from build123d import *

# Parameters (mm, degrees)
SKETCH1_W            = 73.66
SKETCH1_H            = 69.85
BOSS_EXTRUDE1_DEPTH  = 8.89
SKETCH2_R            = 2.032
CUT_EXTRUDE1_DEPTH   = 8.89
SKETCH3_W            = 73.66
SKETCH3_H            = 6.35
BOSS_EXTRUDE2_DEPTH  = 127
SKETCH4_W            = 73.66
SKETCH4_H            = 6.35
BOSS_EXTRUDE3_DEPTH  = 38.1
BOSS_EXTRUDE4_START  = -36.83
BOSS_EXTRUDE4_DEPTH  = 6.35
SKETCH7_R            = 2.54
SKETCH7_R_2          = 6.35
CUT_EXTRUDE2_DEPTH   = 6.35
BOSS_EXTRUDE15_DEPTH = 12.7
SKETCH23_R           = 6.35
BOSS_EXTRUDE16_DEPTH = 6.35
BOSS_EXTRUDE17_DEPTH = 12.7
SKETCH25_W           = 27.94
SKETCH25_H           = 6.35
BOSS_EXTRUDE18_DEPTH = 6.35


with BuildPart() as part:
    # Sketch1 → Boss-Extrude1 (new body)
    with BuildSketch(Plane.XY):
        Rectangle(SKETCH1_W, SKETCH1_H)
    extrude(amount=BOSS_EXTRUDE1_DEPTH)

    # Sketch2 → Cut-Extrude1 (cut)
    with BuildSketch(Plane(origin=(0, 0, 0), x_dir=(-1, 0, 0), z_dir=(0, 0, -1))):
        with Locations((-29.9085, 26.035)):
            Circle(SKETCH2_R)
        with Locations((-29.9085, 8.255)):
            Circle(SKETCH2_R)
        with Locations((29.9085, 8.255)):
            Circle(SKETCH2_R)
        with Locations((29.9085, 26.035)):
            Circle(SKETCH2_R)
    extrude(amount=-CUT_EXTRUDE1_DEPTH, mode=Mode.SUBTRACT)

    # Sketch3 → Boss-Extrude2 (add)
    with BuildSketch(Plane(origin=(0, 0, 0), x_dir=(-1, 0, 0), z_dir=(0, 0, -1))):
        with Locations((0, -31.75)):
            Rectangle(SKETCH3_W, SKETCH3_H)
    extrude(amount=BOSS_EXTRUDE2_DEPTH)

    # Sketch4 → Boss-Extrude3 (add)
    with BuildSketch(Plane.XY.offset(8.89)):
        with Locations((0, -31.75)):
            Rectangle(SKETCH4_W, SKETCH4_H)
    extrude(amount=BOSS_EXTRUDE3_DEPTH)

    # Sketch5 → Boss-Extrude4 (add, symmetric)
    with BuildSketch(Plane(origin=(36.83, 0, 0), x_dir=(0, 0, -1), z_dir=(1, 0, 0)).offset(BOSS_EXTRUDE4_START)):
        Polygon((-46.99, -28.575), (-8.89, 25.837439057), (-8.89, -28.575), align=None)
    extrude(amount=BOSS_EXTRUDE4_DEPTH, both=True)

    # Sketch7 → Cut-Extrude2 (cut)
    with BuildSketch(Plane(origin=(0, -28.575, 0), x_dir=(1, 0, 0), z_dir=(0, 1, 0))):
        with Locations((0, 26.416)):
            Circle(SKETCH7_R)
        with Locations((0, 89.916)):
            Circle(SKETCH7_R_2)
    extrude(amount=-CUT_EXTRUDE2_DEPTH, mode=Mode.SUBTRACT)

    # Sketch21 → Boss-Extrude15 (add)
    with BuildSketch(Plane.ZY.offset(36.83)):
        Polygon((-25.4, -28.575), (-55.626, 3.175), (-49.276, 3.175), (-49.276, 9.525), (-13.0048, -28.575), align=None)
    extrude(amount=-BOSS_EXTRUDE15_DEPTH)

    # Sketch23 → Boss-Extrude16 (add)
    with BuildSketch(Plane(origin=(0, 3.175, 0), x_dir=(1, 0, 0), z_dir=(0, 1, 0))):
        with BuildLine():
            Line((-36.83, 49.276), (8.89, 49.276))
            Line((8.89, 49.276), (8.89, 89.916))
            ThreePointArc((8.89, 89.916), (0, 98.806), (-8.89, 89.916))
            Line((-8.89, 89.916), (-8.89, 55.626))
            Line((-8.89, 55.626), (-36.83, 55.626))
            Line((-36.83, 55.626), (-36.83, 49.276))
        make_face()
        with Locations((0, 89.916)):
            Circle(SKETCH23_R, mode=Mode.SUBTRACT)
    extrude(amount=BOSS_EXTRUDE16_DEPTH)

    # Sketch24 → Boss-Extrude17 (add)
    with BuildSketch(Plane(origin=(36.83, 0, 0), x_dir=(0, 0, -1), z_dir=(1, 0, 0))):
        Polygon((25.4, -28.575), (55.626, 3.175), (49.276, 3.175), (49.276, 9.525), (13.0048, -28.575), align=None)
    extrude(amount=-BOSS_EXTRUDE17_DEPTH)

    # Sketch25 → Boss-Extrude18 (add)
    with BuildSketch(Plane(origin=(0, 3.175, 0), x_dir=(1, 0, 0), z_dir=(0, 1, 0))):
        with Locations((22.86, 52.451)):
            Rectangle(SKETCH25_W, SKETCH25_H)
    extrude(amount=BOSS_EXTRUDE18_DEPTH)


solid = part.part
Design review of the part built by this model. Coordinates are the model's own, in mm. A direction names the side the tool comes from. Round coordinates to 2 decimals unless told otherwise and drop trailing zeros. Write each loop counter-clockwise with the first axis right and the second up, starting at its lowest first coordinate (ties: lowest second). Pieces come first, ordered by that corner, then holes. Notation, with made-up numbers: (70.5, -24) -> (105.5, -24) arc R16 cw to (105.5, -14) -> close; hole circle Ø10 at (-11, 33). An arc over 180 degrees is marked (long way). One line per question, with ' | ' between items.
(1) Insertion check: P1, Ø2.5, axis at x = 29.91, y = 26.04, coming from the -Z side; P2, Ø5.5, axis at x = 29.91, y = 8.26, coming from the -Z side; P3, Ø6.5, axis at x = -29.91, y = 26.04, coming from the -Z side; P4, Ø1.5, axis at x = 5.5, y = 6.5, coming from the -Z side. Each pin has a flat end and moves straight along its axis. Give the tip position at first contact, or say it passes through.
Result sheet:
P1: through | P2: z = -55.63 | P3: z = 0 | P4: z = -97.43
(2) Take a section at C-C, the plane y = -3. State the section outline as (x, z) points.
Result sheet:
outline: (-36.83, -49.75) -> (-24.13, -49.75) -> (-24.13, -37.35) -> (-36.83, -37.35) -> close; (-36.83, 0) -> (36.83, 0) -> (36.83, 8.89) -> (6.35, 8.89) -> (6.35, 29.08) -> (-6.35, 29.08) -> (-6.35, 8.89) -> (-36.83, 8.89) -> close; (24.13, -49.75) -> (36.83, -49.75) -> (36.83, -37.35) -> (24.13, -37.35) -> close
(3) Machinability: for faces 4 (the flat face through (23, 6, -55.626)), 5 (the flat face through (-1, 4, 0)), 6 (the flat face through (6.35, -13, 19)), 7 (the flat face through (-22, -28.575, 28)), 8 (the cylindrical face through (-31.847, 8.865, 4.383)), which of the approach directions +Z, -Z, +X, -X, +Y, -Y give a long, thin tool a straight path to every point of the face, cutting with its end or side? Answer none if there is none.
Result sheet:
face 4: -Z, +X, +Y | face 5: +X, -X, +Y | face 6: +Z, +X, +Y | face 7: +Z, -X, +Y | face 8: +Z
(4) Wall thickness on line 1 (Z direction, x = 0, y = -30.25); line 2 (Z direction, x = 0, y = 8.25); line 3 (Y direction, x = 7.5, z = -3) (3 decimals): over which ranges is each line inside the solid? List them lowest first. Write a range as [from, to].
Result sheet:
line 1: [-127, -96.27], [-83.57, -28.96], [-23.88, 46.99] | line 2: [-98.81, -96.27], [-83.57, -49.28], [0, 21.2] | line 3: [-34.925, -28.575]
(5) Take a section at A-A, the plane z = -61. State the section outline as (x, y) points (3 decimals).
Result sheet:
outline: (-36.83, -34.925) -> (36.83, -34.925) -> (36.83, -28.575) -> (-36.83, -28.575) -> close; (-8.89, 3.175) -> (8.89, 3.175) -> (8.89, 9.525) -> (-8.89, 9.525) -> close
(6) Take a section at D-D, the plane x = -22.5. State the section outline as (y, z) points (3 decimals), and give its area (3 significant figures).
Result sheet:
outline: (-34.925, -127) -> (-28.575, -127) -> (-28.575, 0) -> (34.925, 0) -> (34.925, 8.89) -> (-28.575, 8.89) -> (-28.575, 46.99) -> (-34.925, 46.99) -> close; (3.175, -55.626) -> (9.525, -55.626) -> (9.525, -49.276) -> (3.175, -49.276) -> close | area: 1,710 mm2
(7) Take a section at B-B, the plane x = 0. State the section outline as (y, z) points (3 decimals).
Result sheet:
outline: (-34.925, -127) -> (-28.575, -127) -> (-28.575, -96.266) -> (-34.925, -96.266) -> close; (-34.925, -83.566) -> (-28.575, -83.566) -> (-28.575, -28.956) -> (-34.925, -28.956) -> close; (-34.925, -23.876) -> (-28.575, -23.876) -> (-28.575, 0) -> (34.925, 0) -> (34.925, 8.89) -> (25.837, 8.89) -> (-28.575, 46.99) -> (-34.925, 46.99) -> close; (3.175, -98.806) -> (9.525, -98.806) -> (9.525, -96.266) -> (3.175, -96.266) -> close; (3.175, -83.566) -> (9.525, -83.566) -> (9.525, -49.276) -> (3.175, -49.276) -> close
(8) Draft analysis for pull direction Z (two halves, no side actions). For faces 1 (the flat face through (8, 4, 8.89)), 2 (the cylindrical face through (0.195, 6.306, -98.804)), 3 (the flat face through (-30.57, -9.26, -31.39)), state which applies: released by +Z, released by -Z, zero draft, split by the parting line, or undercut.
Result sheet:
face 1: released by +Z | face 2: released by -Z | face 3: undercut
